```python
from build123d import *

# Parameters (mm, degrees)
F0_W     = 126
F0_H     = 126
F0_W_2   = 120
F0_H_2   = 120
F0_R     = 50
F0_W_3   = 50
F1_DEPTH = 4
F2_DEPTH = 2
F3_R     = 5
F4_W     = 50
F4_H     = 3
F5_DEPTH = 20
F6_W     = 50
F6_H     = 1.5
F6_H_2   = 3
F7_DEPTH = 3
F9_DEPTH = 50
F10_SIZE = 3


with BuildPart() as f1:
    # F0 (on Top) → F1 (new body)
    with BuildSketch(Plane.XY):
        Rectangle(F0_W, F0_H)
        Rectangle(F0_W_2, F0_H_2, mode=Mode.SUBTRACT)
        Rectangle(F0_W_2, F0_H_2)
        Circle(F0_R, mode=Mode.SUBTRACT)
        with Locations((-88, 0)):
            Rectangle(F0_W_3, F0_H)
        with BuildLine():
            Line((-86.25, 48.25), (-86.25, -48.25))
            ThreePointArc((-86.25, -48.25), (-88, -50), (-89.75, -48.25))
            Line((-89.75, -48.25), (-89.75, 48.25))
            ThreePointArc((-89.75, 48.25), (-88, 50), (-86.25, 48.25))
        make_face(mode=Mode.SUBTRACT)
    extrude(amount=F1_DEPTH)

    # F0 (on Top) → F2 (join)
    with BuildSketch(Plane.XY):
        Rectangle(F0_W, F0_H)
        Rectangle(F0_W_2, F0_H_2, mode=Mode.SUBTRACT)
        Rectangle(F0_W_2, F0_H_2)
        Circle(F0_R, mode=Mode.SUBTRACT)
    extrude(amount=-F2_DEPTH)

    # F3
    f3_edges = [f1.edges().sort_by_distance(p)[0] for p in [
        (-113, 63, 2),
        (-113, -63, 2),
        (63, 63, 1),
        (63, -63, 1),
    ]]
    fillet(f3_edges, radius=F3_R)

    # F4 (on face) → F5 (join)
    with BuildSketch(Plane(origin=(0, 0, -2), x_dir=(1, 0, 0), z_dir=(0, 0, -1))):
        with Locations((0, 61.5)):
            Rectangle(F4_W, F4_H)
        with Locations((0, -61.5)):
            Rectangle(F4_W, F4_H)
    extrude(amount=F5_DEPTH)

    # F6 (on face) → F7 (join)
    with BuildSketch(Plane(origin=(0, 0, -22), x_dir=(1, 0, 0), z_dir=(0, 0, -1))):
        Polygon((-25, 60), (-25, 58.5), (25, 58.5), (25, 60), (25, 63), (-25, 63), align=None)
        with Locations((0, -59.25)):
            Rectangle(F6_W, F6_H)
        with Locations((0, -61.5)):
            Rectangle(F6_W, F6_H_2)
    extrude(amount=F7_DEPTH)

    # F8 (on face) → F9 (cut, through all)
    with BuildSketch(Plane.YZ.offset(25)):
        Polygon((-58.5, -25), (-58.5, -22), (-63, -25), align=None)
        Polygon((63, -25), (58.5, -22), (58.5, -25), align=None)
    extrude(amount=-F9_DEPTH, mode=Mode.SUBTRACT)

    # F10
    f10_edges = [f1.edges().sort_by_distance(p)[0] for p in [
        (-50, 0, -2),
    ]]
    chamfer(f10_edges, length=F10_SIZE)


solid = f1.part
```
Model file for the job. Use its own axes, mm. A direction names the side the tool comes from. Give positions to 0.01 mm unless a question says otherwise; leave off trailing zeros. Loops run counter-clockwise (first coordinate to the right, second up) from the corner with the lowest first, then second, coordinate; pieces in that order, holes last. Notation, with made-up numbers: (43.25, 65) -> (49.25, 65) arc R22 ccw to (49.25, 76) -> close; hole circle Ø7 at (36.25, 71.25). An arc over 180 degrees is marked (long way). Use CSV: the item, a comma, the result in double quotes. Start each with the question number.
1) Mould opens along Z. For faces 5 (the flat face through (-86.25, 1, 2)), 6 (the flat face through (0.35, -60.72, -23.48)), 7 (the flat face through (0, 60, -12)) say: released by +Z, released by -Z, zero draft, split by the parting line, or undercut.
2) Wall check: line 1 (X direction, y = 0, z = 3.4); line 2 (Y direction, x = 0, z = 2.75); line 3 (Y direction, x = 18, z = -6). Give the ranges that are in metal, low to high.
3) Slice it at B-B on x = -88. Give the cut face in (y, z), plus the area to 3 significant figures.
4) Flat gauge pins, fed straight in: pin 1 Ø4 at (x, y) = (27.5, -41.5) entering from +Z; pin 2 Ø3.5 at (y, z) = (-61, -13) entering from +X; pin 3 Ø1.6 at (y, z) = (26.5, -1) entering from -X; pin 4 Ø2 at (y, z) = (61.5, -17.5) entering from -X. Where does each tip first touch, or does it go through?
5) Slice it at D-D on x = -66.5. Give the cut face in (y, z).
6) Tool access for faces 1 (the flat face through (25, -62, -13)), 2 (the cylindrical face through (-112, -61, 2)), 3 (the cylindrical face through (-88, 50, 2)), 4 (the flat face through (-25, 62, -13)): list every direction of +Z, -Z, +X, -X, +Y, -Y with a clear straight run to the whole face (end or side of a thin tool).
7) Slice it at A-A on z = -9. Give the cut face in (x, y), plus the area to 3 significant figures.
8) Slice it at C-C on y = 0. Give the number of separate pieces and of enclosed holes in the cut face, plus the area to 3 significant figures.
Computed values:
1,face 5,"zero draft"
1,face 6,"released by -Z"
1,face 7,"undercut"
2,line 1,"x = -113 to -89.75, -86.25 to -50, 50 to 63"
2,line 2,"y = -63 to -50, 50 to 63"
2,line 3,"y = -63 to -60, 60 to 63"
3,outline,"(-63, 0) -> (-50, 0) -> (-50, 4) -> (-63, 4) -> close; (50, 0) -> (63, 0) -> (63, 4) -> (50, 4) -> close"
3,area,"104 mm^2"
4,pin 1,"stops at z = 4"
4,pin 2,"stops at x = 25"
4,pin 3,"stops at x = -63"
4,pin 4,"stops at x = -25"
5,outline,"(-63, 0) -> (63, 0) -> (63, 4) -> (-63, 4) -> close"
6,face 1,"-Z, +X, +Y, -Y"
6,face 2,"+Z, -Z, -X, -Y"
6,face 3,"+Z, -Z"
6,face 4,"-Z, -X, +Y, -Y"
7,outline,"(-25, -63) -> (25, -63) -> (25, -60) -> (-25, -60) -> close; (-25, 60) -> (25, 60) -> (25, 63) -> (-25, 63) -> close"
7,area,"300 mm^2"
8,separate pieces,"3"
8,enclosed holes,"0"
8,area,"333 mm^2"
